```python
from build123d import *

# Parameters (mm, degrees)
F1_DEPTH = 14
F2_DEPTH = 60


with BuildPart() as f1:
    # F0 (on Top) → F1 (new body)
    with BuildSketch(Plane.XY):
        Polygon((0, 14), (0, 0), (45, 0), (45, 14), (43, 14), (43, 12), (43, 2), (33, 2), (2, 2), (2, 4), (2, 12), (2, 14), align=None)
        Polygon((0, 32), (0, 14), (2, 14), (2, 30), (33, 30), (41, 30), (43, 30), (43, 14), (45, 14), (45, 32), align=None)
        with BuildLine():
            Line((23.2020410745, 14), (2, 14))
            Line((2, 14), (2, 12))
            Line((2, 12), (23.0000000447, 12))
            ThreePointArc((23.0000000447, 12), (23.0506385149, 13.0050896201), (23.2020410745, 14))
        make_face()
        with BuildLine():
            Line((2, 30), (2, 14))
            Line((2, 14), (23.2020410745, 14))
            ThreePointArc((23.2020410745, 14), (26.6754447115, 19.7459666607), (33, 21.9999999553))
            Line((33, 21.9999999553), (33, 30))
            Line((33, 30), (2, 30))
        make_face()
        with BuildLine():
            Line((42.7979589255, 14), (43, 14))
            Line((43, 14), (43, 30))
            Line((43, 30), (41, 30))
            Line((41, 30), (41, 17.9999999255))
            ThreePointArc((41, 17.9999999255), (42.1209558342, 16.0997760642), (42.7979589255, 14))
        make_face()
        with BuildLine():
            Line((43, 12), (43, 14))
            Line((43, 14), (42.7979589255, 14))
            ThreePointArc((42.7979589255, 14), (42.9493614851, 13.0050896201), (42.9999999553, 12))
        make_face()
        with BuildLine():
            Line((23.0000000447, 12), (2, 12))
            Line((2, 12), (2, 4))
            Line((2, 4), (27.0000000745, 4))
            ThreePointArc((27.0000000745, 4), (24.0557281433, 7.5278640383), (23.0000000447, 12))
        make_face()
        with BuildLine():
            Line((25.2540333076, 14), (23.2020410745, 14))
            ThreePointArc((23.2020410745, 14), (23.0506385149, 13.0050896201), (23.0000000447, 12))
            Line((23.0000000447, 12), (25, 12))
            ThreePointArc((25, 12), (25.0637624299, 13.0080343399), (25.2540333076, 14))
        make_face()
        with BuildLine():
            ThreePointArc((33, 21.9999999553), (26.6754447115, 19.7459666607), (23.2020410745, 14))
            Line((23.2020410745, 14), (25.2540333076, 14))
            ThreePointArc((25.2540333076, 14), (28.1010205144, 18.3245553203), (33, 20))
            Line((33, 20), (33, 21.9999999553))
        make_face()
        with BuildLine():
            ThreePointArc((41, 6.0000000745), (42.4868329475, 8.8377223822), (42.9999999553, 12))
            ThreePointArc((42.9999999553, 12), (42.9493614851, 13.0050896201), (42.7979589255, 14))
            Line((42.7979589255, 14), (41, 14))
            Line((41, 14), (41, 12))
            Line((41, 12), (41, 6.0000000745))
        make_face()
        with BuildLine():
            Line((43, 2), (43, 12))
            ThreePointArc((42.9999999553, 12), (42.4868329475, 8.8377223822), (41, 6.0000000745))
            Line((41, 6.0000000745), (41, 4))
            Line((41, 4), (38.9999999255, 4))
            ThreePointArc((38.9999999255, 4), (36.1622776178, 2.5131670525), (33, 2.0000000447))
            Line((33, 2), (43, 2))
        make_face()
        with BuildLine():
            Line((41, 14), (42.7979589255, 14))
            ThreePointArc((42.7979589255, 14), (42.1209558342, 16.0997760642), (41, 17.9999999255))
            Line((41, 17.9999999255), (41, 14))
        make_face()
        with BuildLine():
            Line((27.0000000745, 4), (2, 4))
            Line((2, 4), (2, 2))
            Line((2, 2), (33, 2))
            ThreePointArc((33, 2.0000000447), (29.8377223822, 2.5131670525), (27.0000000745, 4))
        make_face()
        with BuildLine():
            Line((25, 12), (23.0000000447, 12))
            ThreePointArc((23.0000000447, 12), (24.0557281433, 7.5278640383), (27.0000000745, 4))
            Line((27.0000000745, 4), (33, 4))
            ThreePointArc((33, 4), (27.3431457505, 6.3431457505), (25, 12))
        make_face()
        with BuildLine():
            Line((41, 30), (33, 30))
            Line((33, 30), (33, 21.9999999553))
            ThreePointArc((33, 21.9999999553), (37.4721359617, 20.9442718567), (41, 17.9999999255))
            Line((41, 17.9999999255), (41, 30))
        make_face()
        with BuildLine():
            ThreePointArc((38.9999999255, 4), (40.0710677803, 4.9289322197), (41, 6.0000000745))
            Line((41, 6.0000000745), (41, 12))
            ThreePointArc((41, 12), (38.6568542495, 6.3431457505), (33, 4))
            Line((33, 4), (38.9999999255, 4))
        make_face()
        with BuildLine():
            Line((41, 4), (41, 6.0000000745))
            ThreePointArc((41, 6.0000000745), (40.0710677803, 4.9289322197), (38.9999999255, 4))
            Line((38.9999999255, 4), (41, 4))
        make_face()
        with BuildLine():
            Line((41, 12), (41, 14))
            Line((41, 14), (40.7459666924, 14))
            ThreePointArc((40.7459666924, 14), (40.9362375701, 13.0080343399), (41, 12))
        make_face()
        with BuildLine():
            Line((33, 4), (27.0000000745, 4))
            ThreePointArc((27.0000000745, 4), (29.8377223822, 2.5131670525), (33, 2.0000000447))
            ThreePointArc((33, 2.0000000447), (36.1622776178, 2.5131670525), (38.9999999255, 4))
            Line((38.9999999255, 4), (33, 4))
        make_face()
    extrude(amount=F1_DEPTH)

    # F0 (on Top) → F2 (join)
    with BuildSketch(Plane.XY):
        with BuildLine():
            Line((25.2540333076, 14), (23.2020410745, 14))
            ThreePointArc((23.2020410745, 14), (23.0506385149, 13.0050896201), (23.0000000447, 12))
            Line((23.0000000447, 12), (25, 12))
            ThreePointArc((25, 12), (25.0637624299, 13.0080343399), (25.2540333076, 14))
        make_face()
        with BuildLine():
            ThreePointArc((33, 21.9999999553), (26.6754447115, 19.7459666607), (23.2020410745, 14))
            Line((23.2020410745, 14), (25.2540333076, 14))
            ThreePointArc((25.2540333076, 14), (28.1010205144, 18.3245553203), (33, 20))
            Line((33, 20), (33, 21.9999999553))
        make_face()
        with BuildLine():
            ThreePointArc((41, 6.0000000745), (42.4868329475, 8.8377223822), (42.9999999553, 12))
            ThreePointArc((42.9999999553, 12), (42.9493614851, 13.0050896201), (42.7979589255, 14))
            Line((42.7979589255, 14), (41, 14))
            Line((41, 14), (41, 12))
            Line((41, 12), (41, 6.0000000745))
        make_face()
        with BuildLine():
            Line((41, 14), (42.7979589255, 14))
            ThreePointArc((42.7979589255, 14), (42.1209558342, 16.0997760642), (41, 17.9999999255))
            Line((41, 17.9999999255), (41, 14))
        make_face()
        with BuildLine():
            Line((25, 12), (23.0000000447, 12))
            ThreePointArc((23.0000000447, 12), (24.0557281433, 7.5278640383), (27.0000000745, 4))
            Line((27.0000000745, 4), (33, 4))
            ThreePointArc((33, 4), (27.3431457505, 6.3431457505), (25, 12))
        make_face()
        with BuildLine():
            ThreePointArc((41, 17.9999999255), (37.4721359617, 20.9442718567), (33, 21.9999999553))
            Line((33, 21.9999999553), (33, 20))
            ThreePointArc((33, 20), (37.8989794856, 18.3245553203), (40.7459666924, 14))
            Line((40.7459666924, 14), (41, 14))
            Line((41, 14), (41, 17.9999999255))
        make_face()
        with BuildLine():
            ThreePointArc((38.9999999255, 4), (40.0710677803, 4.9289322197), (41, 6.0000000745))
            Line((41, 6.0000000745), (41, 12))
            ThreePointArc((41, 12), (38.6568542495, 6.3431457505), (33, 4))
            Line((33, 4), (38.9999999255, 4))
        make_face()
        with BuildLine():
            Line((41, 12), (41, 14))
            Line((41, 14), (40.7459666924, 14))
            ThreePointArc((40.7459666924, 14), (40.9362375701, 13.0080343399), (41, 12))
        make_face()
        with BuildLine():
            Line((33, 4), (27.0000000745, 4))
            ThreePointArc((27.0000000745, 4), (29.8377223822, 2.5131670525), (33, 2.0000000447))
            ThreePointArc((33, 2.0000000447), (36.1622776178, 2.5131670525), (38.9999999255, 4))
            Line((38.9999999255, 4), (33, 4))
        make_face()
    extrude(amount=F2_DEPTH)


solid = f1.part
```
Geometry: final body of the model. Coordinates: model frame, mm. Give positions to 0.01 mm unless a question says otherwise; leave off trailing zeros. Loops run counter-clockwise (first coordinate to the right, second up) from the corner with the lowest first, then second, coordinate; pieces in that order, holes last. Notation, with made-up numbers: (17.5, 50) -> (62.5, 50) arc R14 ccw to (62.5, 63) -> close; hole circle Ø6 at (18, -30.5). An arc over 180 degrees is marked (long way). Use one line per item in the form item = value.
Item 1: Section query B-B on y = 15.5. Output: boundary loops of the cut face in (x, z).
A:
outline = (0, 0) -> (25.81, 0) -> (25.81, 60) -> (23.63, 60) -> (23.63, 14) -> (0, 14) -> close; (40.19, 0) -> (45, 0) -> (45, 14) -> (42.37, 14) -> (42.37, 60) -> (40.19, 60) -> close
Item 2: Pin query (flat end, axial travel): P1, Ø3, axis at y = 22, z = 41, coming from the +X side; P2, Ø1, axis at x = 31, z = 33, coming from the +Y side; P3, Ø2, axis at x = 23.5, z = 17, coming from the -Y side; P4, Ø1.5, axis at x = 7, z = 15, coming from the +Y side. Return the tip coordinate at first contact, or that it passes through.
A:
P1 = 38.27
P2 = 21.89
P3 = 6.73
P4 = through
Item 3: Section query C-C on y = 3. Output: boundary loops of the cut face in (x, z).
A:
outline = (0, 0) -> (45, 0) -> (45, 14) -> (37.36, 14) -> (37.36, 60) -> (28.64, 60) -> (28.64, 14) -> (0, 14) -> close
Item 4: Line query: probe 1 along Y at (x, z) = (33, 17); probe 2 along X at (y, z) = (12, 23); probe 3 along Z at (x, y) = (4, 17). Output: solid intervals per line, ascending.
A:
probe_1 = 2 to 4, 20 to 22
probe_2 = 23 to 25, 41 to 43
probe_3 = 0 to 14
Item 5: Draft query along Y for faces 1 (the face through (41, 12, 30)), 2 (the face through (22, 0, 7)), 3 (the face through (45, 16, 7)). Return one class per face: pulls with the +Y half, pulls with the -Y half, needs draft (parallel to the pull), parting line crosses it, or undercut.
A:
face_1 = undercut
face_2 = pulls with the -Y half
face_3 = needs draft
Item 6: Section query A-A on z = 28.5. Output: boundary loops of the cut face in (x, y).
A:
outline = circle Ø20 at (33, 12); hole circle Ø16 at (33, 12)
Item 7: Section query D-D on z = 5. Output: boundary loops of the cut face in (x, y).
A:
outline = (0, 0) -> (45, 0) -> (45, 32) -> (0, 32) -> close; hole circle Ø16 at (33, 12)
